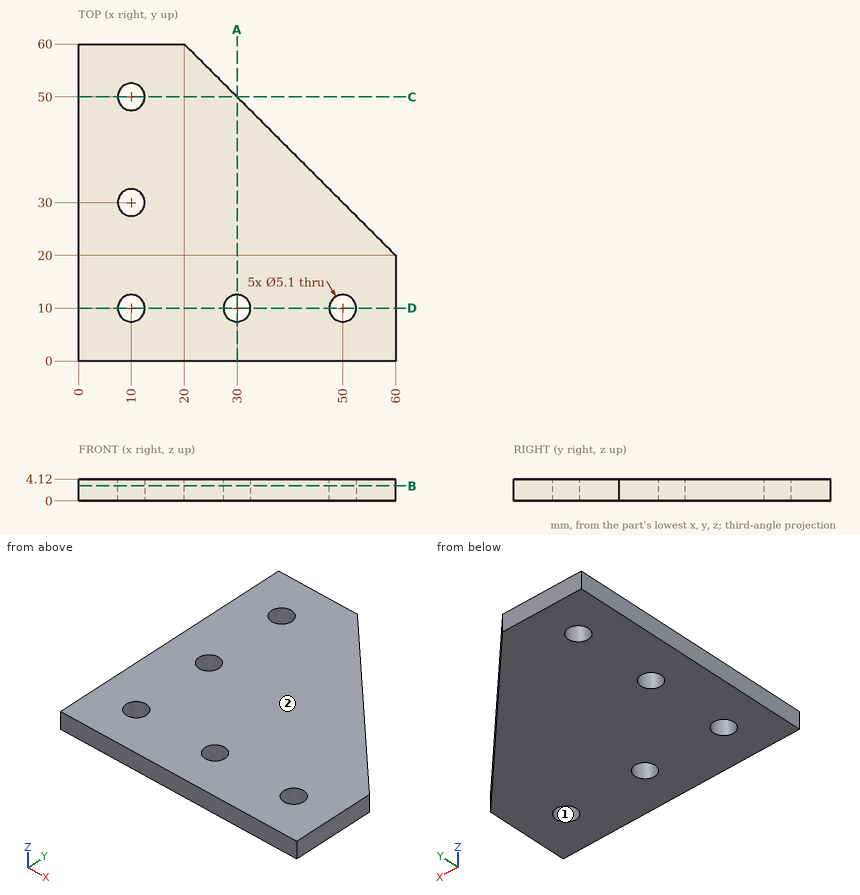
Source: three-view drawing plus pictorial views. Frame: mm from the lowest corner of the part. Coordinates: 2 decimals unless noted, no trailing zeros. Write each loop counter-clockwise with the first axis right and the second up, starting at its lowest first coordinate (ties: lowest second). Pieces come first, ordered by that corner, then holes. Notation, with made-up numbers: (23, 73.5) -> (44, 73.5) arc R26 cw to (44, 99.5) -> close; hole circle Ø6 at (83.5, 30). An arc over 180 degrees is marked (long way). Answer as a JSON object with one key per item and string values.
1. Section A-A on x = 30. Return the cut outline in (y, z), then the cut area to 3 significant figures.
Result set:
{"outline": "(0, 0) -> (7.45, 0) -> (7.45, 4.12) -> (0, 4.12) -> close; (12.55, 0) -> (50, 0) -> (50, 4.12) -> (12.55, 4.12) -> close", "area": "185 mm2"}
2. Section D-D on y = 10. Return the cut outline in (x, z), then the cut area to 3 significant figures.
Result set:
{"outline": "(0, 0) -> (7.45, 0) -> (7.45, 4.12) -> (0, 4.12) -> close; (12.55, 0) -> (27.45, 0) -> (27.45, 4.12) -> (12.55, 4.12) -> close; (32.55, 0) -> (47.45, 0) -> (47.45, 4.12) -> (32.55, 4.12) -> close; (52.55, 0) -> (60, 0) -> (60, 4.12) -> (52.55, 4.12) -> close", "area": "184 mm2"}
3. Material intervals for line 1 (Y direction, x = 10, z = 1.8); line 2 (Y direction, x = 50, z = 1.55); line 3 (X direction, y = 31.5, z = 1.3), sorted ascending. Write a range as from..to.
Result set:
{"line 1": "y = 0..7.45, 12.55..27.45, 32.55..47.45, 52.55..60", "line 2": "y = 0..7.45, 12.55..30", "line 3": "x = 0..7.94, 12.06..48.5"}
4. Section C-C on y = 50. Return the cut outline in (x, z).
Result set:
{"outline": "(0, 0) -> (7.45, 0) -> (7.45, 4.12) -> (0, 4.12) -> close; (12.55, 0) -> (30, 0) -> (30, 4.12) -> (12.55, 4.12) -> close"}
5. Section B-B on z = 2.8. Return the cut outline in (x, y).
Result set:
{"outline": "(0, 0) -> (60, 0) -> (60, 20) -> (20, 60) -> (0, 60) -> close; hole circle Ø5.1 at (10, 10); hole circle Ø5.1 at (10, 30); hole circle Ø5.1 at (10, 50); hole circle Ø5.1 at (30, 10); hole circle Ø5.1 at (50, 10)"}
6. Mould query, pull axis Y, two halves, no side actions, for the marked faces 1 and 2. Classes: released by +Y, released by -Y, zero draft, split by the parting line, or undercut.
Result set:
{"face 1": "undercut", "face 2": "zero draft"}
